Verification items for this drawing (mm, ordinates from the low corner). Give positions to 0.01 mm unless a question says otherwise; leave off trailing zeros. Write each loop counter-clockwise with the first axis right and the second up, starting at its lowest first coordinate (ties: lowest second). Pieces come first, ordered by that corner, then holes. Notation, with made-up numbers: (85.25, 79.5) -> (134.25, 79.5) arc R14 ccw to (134.25, 89.5) -> close; hole circle Ø1 at (-29.5, 42). An arc over 180 degrees is marked (long way). One line per item, written item: value.
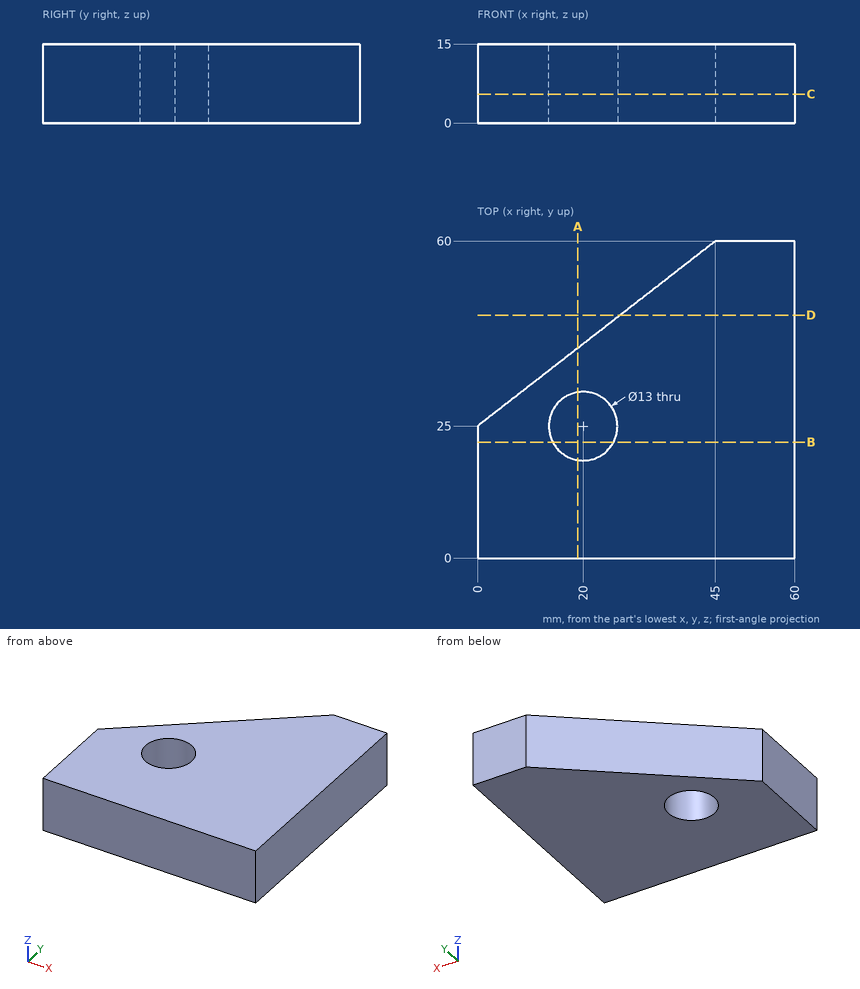
1) Sectioned sample at B-B on y = 22. Record the cut outline in (x, z).
Verdict:
outline: (0, 0) -> (14.23, 0) -> (14.23, 15) -> (0, 15) -> close; (25.77, 0) -> (60, 0) -> (60, 15) -> (25.77, 15) -> close
2) Sectioned sample at A-A on x = 19. Record the cut outline in (y, z).
Verdict:
outline: (0, 0) -> (18.58, 0) -> (18.58, 15) -> (0, 15) -> close; (31.42, 0) -> (39.78, 0) -> (39.78, 15) -> (31.42, 15) -> close
3) Sectioned sample at C-C on z = 5.5. Record the cut outline in (x, y), plus the area to 3 significant figures.
Verdict:
outline: (0, 0) -> (60, 0) -> (60, 60) -> (45, 60) -> (0, 25) -> close; hole circle Ø13 at (20, 25)
area: 2,680 mm^2
4) Depth check by flat-ended pin: pin 1 Ø2 at (y, z) = (46.5, 13) entering from -X. Enter the tip coordinate at first touch or a pass-through.
Verdict:
pin 1: x = 26.36
5) Scan lines: probe 1 along Y at (x, z) = (20, 9); probe 2 along X at (y, z) = (21, 6.75); probe 3 along Y at (x, z) = (15.5, 5.25). Record each from-to range of solid material in increasing order.
Verdict:
probe 1: 0 to 18.5, 31.5 to 40.56
probe 2: 0 to 14.88, 25.12 to 60
probe 3: 0 to 20.31, 29.69 to 37.06
6) Sectioned sample at D-D on y = 46. Record the cut outline in (x, z).
Verdict:
outline: (27, 0) -> (60, 0) -> (60, 15) -> (27, 15) -> close
